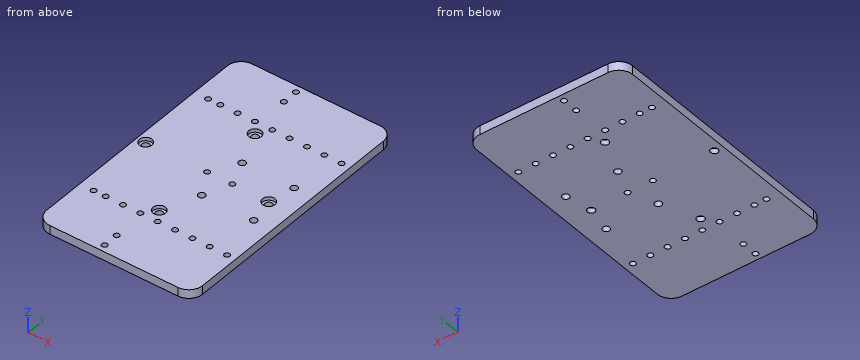
from build123d import *

# Parameters (mm, degrees)
SKETCH_1_W          = 90
SKETCH_1_H          = 150
SKETCH_1_R          = 2
SKETCH_1_R_2        = 2.15
SKETCH_1_R_3        = 1.6
EXTRUDE_1_DEPTH     = 5
FILLET_1_R          = 8
SKETCH_2_R          = 3.6
CUT_EXTRUDE_1_DEPTH = 2


with BuildPart() as part:
    # 草图1 → 凸台-拉伸1 (new body)
    with BuildSketch(Plane.XY):
        with Locations((45, -75)):
            Rectangle(SKETCH_1_W, SKETCH_1_H)
        with Locations((79, -60)):
            Circle(SKETCH_1_R, mode=Mode.SUBTRACT)
        with Locations((79, -90)):
            Circle(SKETCH_1_R, mode=Mode.SUBTRACT)
        with Locations((49, -60)):
            Circle(SKETCH_1_R, mode=Mode.SUBTRACT)
        with Locations((49, -90)):
            Circle(SKETCH_1_R, mode=Mode.SUBTRACT)
        with Locations((40.5, -39.5)):
            Circle(SKETCH_1_R_2, mode=Mode.SUBTRACT)
        with Locations((40.5, -110.5)):
            Circle(SKETCH_1_R_2, mode=Mode.SUBTRACT)
        with Locations((76, -75)):
            Circle(SKETCH_1_R_2, mode=Mode.SUBTRACT)
        with Locations((5, -75)):
            Circle(SKETCH_1_R_2, mode=Mode.SUBTRACT)
        with Locations((85, -117.5)):
            Circle(SKETCH_1_R_3, mode=Mode.SUBTRACT)
        with Locations((75, -117.5)):
            Circle(SKETCH_1_R_3, mode=Mode.SUBTRACT)
        with Locations((65, -117.5)):
            Circle(SKETCH_1_R_3, mode=Mode.SUBTRACT)
        with Locations((55, -117.5)):
            Circle(SKETCH_1_R_3, mode=Mode.SUBTRACT)
        with Locations((45, -117.5)):
            Circle(SKETCH_1_R_3, mode=Mode.SUBTRACT)
        with Locations((85, -32.5)):
            Circle(SKETCH_1_R_3, mode=Mode.SUBTRACT)
        with Locations((75, -32.5)):
            Circle(SKETCH_1_R_3, mode=Mode.SUBTRACT)
        with Locations((65, -32.5)):
            Circle(SKETCH_1_R_3, mode=Mode.SUBTRACT)
        with Locations((55, -32.5)):
            Circle(SKETCH_1_R_3, mode=Mode.SUBTRACT)
        with Locations((45, -32.5)):
            Circle(SKETCH_1_R_3, mode=Mode.SUBTRACT)
        with Locations((35, -117.5)):
            Circle(SKETCH_1_R_3, mode=Mode.SUBTRACT)
        with Locations((25, -117.5)):
            Circle(SKETCH_1_R_3, mode=Mode.SUBTRACT)
        with Locations((15, -117.5)):
            Circle(SKETCH_1_R_3, mode=Mode.SUBTRACT)
        with Locations((35, -32.5)):
            Circle(SKETCH_1_R_3, mode=Mode.SUBTRACT)
        with Locations((25, -32.5)):
            Circle(SKETCH_1_R_3, mode=Mode.SUBTRACT)
        with Locations((15, -32.5)):
            Circle(SKETCH_1_R_3, mode=Mode.SUBTRACT)
        with Locations((8, -117.5)):
            Circle(SKETCH_1_R_3, mode=Mode.SUBTRACT)
        with Locations((8, -32.5)):
            Circle(SKETCH_1_R_3, mode=Mode.SUBTRACT)
        with Locations((36.5, -4)):
            Circle(SKETCH_1_R_3, mode=Mode.SUBTRACT)
        with Locations((36.5, -13)):
            Circle(SKETCH_1_R_3, mode=Mode.SUBTRACT)
        with Locations((36.5, -137)):
            Circle(SKETCH_1_R_3, mode=Mode.SUBTRACT)
        with Locations((36.5, -146)):
            Circle(SKETCH_1_R_3, mode=Mode.SUBTRACT)
        with Locations((55, -75)):
            Circle(SKETCH_1_R_3, mode=Mode.SUBTRACT)
        with Locations((40.5, -75)):
            Circle(SKETCH_1_R_3, mode=Mode.SUBTRACT)
    extrude(amount=EXTRUDE_1_DEPTH)

    # 圆角1
    fillet_1_edges = [part.edges().sort_by_distance(p)[0] for p in [
        (0, 0, 2.5),
        (90, 0, 2.5),
        (90, -150, 2.5),
        (0, -150, 2.5),
    ]]
    fillet(fillet_1_edges, radius=FILLET_1_R)

    # 草图2 → 切除-拉伸1 (cut)
    with BuildSketch(Plane.XY.offset(5)):
        with Locations((40.5, -39.5)):
            Circle(SKETCH_2_R)
        with Locations((76, -75)):
            Circle(SKETCH_2_R)
        with Locations((5, -75)):
            Circle(SKETCH_2_R)
        with Locations((40.5, -110.5)):
            Circle(SKETCH_2_R)
    extrude(amount=-CUT_EXTRUDE_1_DEPTH, mode=Mode.SUBTRACT)


solid = part.part
Read the model definition and answer for the solid it produces. Units are mm, in the model's axes. Round coordinates to 2 decimals unless told otherwise and drop trailing zeros. Order: outer loops, then holes, each group sorted by start corner. A loop starts at its lowest first (then second) coordinate and runs counter-clockwise, first axis right, second up. Notation, with made-up numbers: (73, -21) - (117, -21) arc R23 cw to (117, 9) - close; hole circle Ø8 at (10.5, 1.5). An arc over 180 degrees is marked (long way). Use one line per item in the form item = value. Start each with the question number.
(1) The part is cut by section D-D (y = -60). Give the vertices of the cut face in (x, z), then the cut area to 3 significant figures.
(2) A flat-ended cylindrical pin translates along its axis: pin 1 Ø7 at (x, y) = (76, -75) entering from +Z. Find the tip coordinate at first contact, or state that the pin passes through.
(3) The part is cut by section A-A (y = -137). Give the vertices of the cut face in (x, z), then the cut area to 3 significant figures.
(4) Find the intervals of material crossed by line 1 along Y through (x, z) = (40.5, 4.65); line 2 along Y through (x, z) = (45, 3.8); line 3 along Y through (x, z) = (49.5, 4.85), in increasing order. Write a range as from..to.
(5) The part is cut by section B-B (x = 25). Give the vertices of the cut face in (y, z), then the cut area to 3 significant figures.
(6) The part is cut by section C-C (x = 40.5). Give the vertices of the cut face in (y, z).
Checked values:
q1.outline = (0, 0) - (47, 0) - (47, 5) - (0, 5) - close; (51, 0) - (77, 0) - (77, 5) - (51, 5) - close; (81, 0) - (90, 0) - (90, 5) - (81, 5) - close
q1.area = 410 mm^2
q2.pin_1 = 3
q3.outline = (0, 0) - (34.9, 0) - (34.9, 5) - (0, 5) - close; (38.1, 0) - (90, 0) - (90, 5) - (38.1, 5) - close
q3.area = 434 mm^2
q4.line_1 = -150..-114.1, -106.9..-76.6, -73.4..-43.1, -35.9..0
q4.line_2 = -150..-119.1, -115.9..-34.1, -30.9..0
q4.line_3 = -150..-91.94, -88.06..-61.94, -58.06..0
q5.outline = (-150, 0) - (-119.1, 0) - (-119.1, 5) - (-150, 5) - close; (-115.9, 0) - (-34.1, 0) - (-34.1, 5) - (-115.9, 5) - close; (-30.9, 0) - (0, 0) - (0, 5) - (-30.9, 5) - close
q5.area = 718 mm^2
q6.outline = (-150, 0) - (-112.65, 0) - (-112.65, 3) - (-114.1, 3) - (-114.1, 5) - (-150, 5) - close; (-108.35, 0) - (-76.6, 0) - (-76.6, 5) - (-106.9, 5) - (-106.9, 3) - (-108.35, 3) - close; (-73.4, 0) - (-41.65, 0) - (-41.65, 3) - (-43.1, 3) - (-43.1, 5) - (-73.4, 5) - close; (-37.35, 0) - (0, 0) - (0, 5) - (-35.9, 5) - (-35.9, 3) - (-37.35, 3) - close
